```python
from build123d import *

# Parameters (mm, degrees)
EXTRUDE_1_DEPTH          = 65
EXTRUDE_1_DEPTH_BACK     = 65
SKETCH_1_R               = 23
EXTRUDE_3_DEPTH          = 24
SKETCH_7_R               = 6
CUT_EXTRUDE_3_DEPTH      = 24
SKETCH_8_R               = 21
EXTRUDE_4_DEPTH          = 40
CUT_EXTRUDE_2_DEPTH      = 65
CUT_EXTRUDE_2_DEPTH_BACK = 65
SKETCH_3_R               = 12
CUT_EXTRUDE_1_DEPTH      = 47
CUT_EXTRUDE_1_DEPTH_BACK = 47
SKETCH_2_R               = 15
EXTRUDE_5_DEPTH          = 12
SKETCH_11_R              = 12
SKETCH_11_R_2            = 6
CUT_EXTRUDE_4_DEPTH      = 40


with BuildPart() as part:
    # Sketch 1 → Extrude 1 (new, two sides: drawn at the far end of the back side and taken through both)
    with BuildSketch(Plane(origin=(0, 0, 0), x_dir=(0, 0, -1), z_dir=(1, 0, 0)).offset(-EXTRUDE_1_DEPTH_BACK)):
        Circle(SKETCH_1_R)
    extrude(amount=EXTRUDE_1_DEPTH + EXTRUDE_1_DEPTH_BACK)

    # Sketch 4 → Extrude 3 (add)
    with BuildSketch(Plane(origin=(65, 0, 0), x_dir=(0, 0, -1), z_dir=(1, 0, 0))):
        Polygon((-44.703636651, 33), (-20, 33), (-14, 33), (14, 33), (20, 33), (45.296363349, 33), (45.296363349, 45), (20, 45), (-20, 45), (-44.703636651, 45), align=None)
        Polygon((-20, 33), (-20, 11.357816692), (-14, 18.248287591), (-14, 33), align=None)
        Polygon((14, 33), (14, 18.248287591), (20, 11.357816692), (20, 33), align=None)
    extrude(amount=-EXTRUDE_3_DEPTH)

    # Sketch 7 → Cut-Extrude 3 (cut)
    with BuildSketch(Plane(origin=(0, 45, 0), x_dir=(1, 0, 0), z_dir=(0, 1, 0))):
        with Locations(Location((53, 35, 0), (0, 0, 270))):
            Circle(SKETCH_7_R)
        with Locations(Location((53, -35, 0), (0, 0, 270))):
            Circle(SKETCH_7_R)
    extrude(amount=-CUT_EXTRUDE_3_DEPTH, mode=Mode.SUBTRACT)

    # Sketch 8 → Extrude 4 (add)
    with BuildSketch(Plane.XY):
        with Locations(Location((-43, 0, 0), (0, 0, 180))):
            Circle(SKETCH_8_R)
    extrude(amount=EXTRUDE_4_DEPTH)

    # Sketch 3 → Cut-Extrude 2 (cut, two sides: drawn at the far end of the back side and taken through both)
    with BuildSketch(Plane(origin=(0, 0, 0), x_dir=(0, 0, -1), z_dir=(1, 0, 0)).offset(-CUT_EXTRUDE_2_DEPTH_BACK)):
        Circle(SKETCH_3_R)
    extrude(amount=CUT_EXTRUDE_2_DEPTH + CUT_EXTRUDE_2_DEPTH_BACK, mode=Mode.SUBTRACT)

    # Sketch 2 → Cut-Extrude 1 (cut, two sides: drawn at the far end of the back side and taken through both)
    with BuildSketch(Plane(origin=(0, 0, 0), x_dir=(0, 0, -1), z_dir=(1, 0, 0)).offset(-CUT_EXTRUDE_1_DEPTH_BACK)):
        Circle(SKETCH_2_R)
    extrude(amount=CUT_EXTRUDE_1_DEPTH + CUT_EXTRUDE_1_DEPTH_BACK, mode=Mode.SUBTRACT)

    # Sketch 10 → Extrude 5 (add)
    with BuildSketch(Plane.XY.offset(40)):
        with BuildLine():
            Line((-54.313708499, 37), (-64.684607956, 7.666666667))
            ThreePointArc((-64.684607956, 7.666666667), (-66, 0), (-64.684607956, -7.666666667))
            Line((-64.684607956, -7.666666667), (-54.313708499, -37))
            ThreePointArc((-54.313708499, -37), (-43, -45), (-31.686291501, -37))
            Line((-31.686291501, -37), (-21.315392044, -7.666666667))
            ThreePointArc((-21.315392044, -7.666666667), (-20, 0), (-21.315392044, 7.666666667))
            Line((-21.315392044, 7.666666667), (-31.686291501, 37))
            ThreePointArc((-31.686291501, 37), (-43, 45), (-54.313708499, 37))
        make_face()
    extrude(amount=-EXTRUDE_5_DEPTH)

    # Sketch 11 → Cut-Extrude 4 (cut)
    with BuildSketch(Plane.XY.offset(40)):
        with Locations((-43, 0)):
            Circle(SKETCH_11_R)
        with Locations((-43, 33)):
            Circle(SKETCH_11_R_2)
        with Locations((-43, -33)):
            Circle(SKETCH_11_R_2)
    extrude(amount=-CUT_EXTRUDE_4_DEPTH, mode=Mode.SUBTRACT)


solid = part.part
```
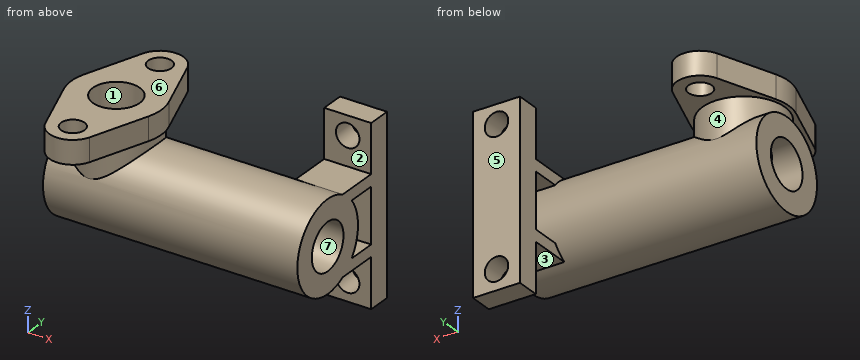
The listing builds one solid part. Answer for the finished solid, in the listing's coordinates (mm). Face numbers are marked on the shaded views. A direction names the side the tool comes from. Round coordinates to 2 decimals unless told otherwise and drop trailing zeros. Write each loop counter-clockwise with the first axis right and the second up, starting at its lowest first coordinate (ties: lowest second). Pieces come first, ordered by that corner, then holes. Notation, with made-up numbers: (20, -10) -> (41, -10) arc R17 ccw to (41, 5) -> close; hole circle Ø7 at (-16.5, 55). An arc over 180 degrees is marked (long way). Answer as a JSON object with one key per item and string values. Group by question number.
Q1. Section C-C (z = 0) is taken. Write down the section's boundary in (x, y), plus the area to 3 significant figures.
Q2. Straight lines are drawn through the part: line 1 along Y through (x, z) = (-43, 30); line 2 along Y through (x, z) = (52, 0); line 3 along Y through (x, z) = (-44.5, 28.5). For each, find the intervals that lie inside material, in ascending order.
Q3. Which of the six approach directions +Z, -Z, +X, -X, +Y, -Y give full straight-line access (tool end or side, diameter ignored) to the marked faces 1, 2, 3 and 4?
Q4. Each of these flat-tipped pins is pushed along its axis until it touches: pin 1 Ø6 at (x, z) = (-37, 12.5) entering from -Y; pin 2 Ø2 at (x, z) = (-24.5, 7) entering from +Y; pin 3 Ø4 at (y, z) = (17.5, -18) entering from -X. Where does it stop, or does it pass through?
Q5. Section B-B (z = 35) is taken. Write down the section's boundary in (x, y).
Q6. Section D-D (x = -43) is taken. Write down the section's boundary in (y, z), plus the area to 3 significant figures.
Q7. Section A-A (x = 53) is taken. Write down the section's boundary in (y, z), plus the area to 3 significant figures.
Q8. Determine the mould class of the marked faces 5, 6 and 7 for opening direction Y: pulls with the +Y half, pulls with the -Y half, needs draft (parallel to the pull), parting line crosses it, or undercut.
Check values:
{
 "1": {"outline": "(-65, -23) -> (65, -23) -> (65, -12) -> (47, -12) -> (47, -15) -> (-47, -15) -> (-47, -12) -> (-65, -12) -> close; (-65, 12) -> (-47, 12) -> (-47, 15) -> (47, 15) -> (47, 12) -> (65, 12) -> (65, 23) -> (-65, 23) -> close; (41, 33) -> (65, 33) -> (65, 45) -> (41, 45) -> close", "area": "2,580 mm^2"},
 "2": {"line 1": "-45 to -39, -27 to -12, 12 to 27, 39 to 45", "line 2": "-23 to -12, 12 to 23, 33 to 45", "line 3": "-44.91 to -38.81, -27.19 to -11.91, 11.91 to 27.19, 38.81 to 44.91"},
 "3": {"face 1": "+Z", "face 2": "+Z, +X", "face 3": "-Z, +X, -X", "face 4": "none"},
 "4": {"pin 1": "y = -20.95", "pin 2": "y = 22.2", "pin 3": "x = 41"},
 "5": {"outline": "(-64.68, -7.67) -> (-54.31, -37) arc R12 ccw to (-31.69, -37) -> (-21.32, -7.67) arc R23 ccw to (-21.32, 7.67) -> (-31.69, 37) arc R12 ccw to (-54.31, 37) -> (-64.68, 7.67) arc R23 ccw to start; (41, 33) -> (47, 33) -> (47, 45) -> (41, 45) -> close; (59, 33) -> (65, 33) -> (65, 45) -> (59, 45) -> close; hole circle Ø24 at (-43, 0); hole circle Ø12 at (-43, -33); hole circle Ø12 at (-43, 33)"},
 "6": {"outline": "(-45, 28) -> (-39, 28) -> (-39, 40) -> (-45, 40) -> close; (-27, 28) -> (-21, 28) -> (-21, 9.38) arc R23 ccw (long way) to (21, 9.38) -> (21, 28) -> (27, 28) -> (27, 40) -> (12, 40) -> (12, 9) arc R15 cw (long way) to (-12, 9) -> (-12, 40) -> (-27, 40) -> close; (39, 28) -> (45, 28) -> (45, 40) -> (39, 40) -> close", "area": "1,470 mm^2"},
 "7": {"outline": "(11.36, -20) -> (33, -20) -> (33, -29) -> (45, -29) -> (45, 29) -> (33, 29) -> (33, 20) -> (11.36, 20) arc R23 ccw (long way) to start; (33, -45.3) -> (45, -45.3) -> (45, -41) -> (33, -41) -> close; (33, 41) -> (45, 41) -> (45, 44.7) -> (33, 44.7) -> close; hole circle Ø24 at (0, 0); hole (18.25, -14) -> (33, -14) -> (33, 14) -> (18.25, 14) arc R23 cw to start", "area": "2,210 mm^2"},
 "8": {"face 5": "pulls with the +Y half", "face 6": "needs draft", "face 7": "undercut"}
}
